```python
from build123d import *

# Parameters (mm, degrees)
F0_W     = 41.78606
F0_H     = 0.478756
F1_DEPTH = 1.5
F0_H_2   = 15.542488
F2_DEPTH = 1
F3_DEPTH = 1.5


with BuildPart() as f1:
    # F0 (on Right) → F1 (new body)
    with BuildSketch(Plane.YZ):
        with Locations((0, -8.010622)):
            Rectangle(F0_W, F0_H)
    extrude(amount=F1_DEPTH)

    # F0 (on Right) → F2 (join)
    with BuildSketch(Plane.YZ):
        with Locations((0, 8.010622)):
            Rectangle(F0_W, F0_H)
        Rectangle(F0_W, F0_H_2)
        with Locations((0, -8.010622)):
            Rectangle(F0_W, F0_H)
    extrude(amount=F2_DEPTH)

    # F0 (on Right) → F3 (join)
    with BuildSketch(Plane.YZ):
        with Locations((0, 8.010622)):
            Rectangle(F0_W, F0_H)
    extrude(amount=F3_DEPTH)


solid = f1.part
```
Design review of the part built by this model. Coordinates are the model's own, in mm. Coordinates: 2 decimals unless noted, no trailing zeros. Order: outer loops, then holes, each group sorted by start corner. A loop starts at its lowest first (then second) coordinate and runs counter-clockwise, first axis right, second up. Notation, with made-up numbers: M 11,-34 L 30,-34 A23 ccw 30,-24 Z; hole C 4,82 d9. An arc over 180 degrees is marked long. Answer as a JSON object with one key per item and string values. Group by question number.
1) Add section B-B, the plane y = -3.5. Write out the cut boundary in (x, z).
2) Add section C-C, the plane z = 7. Write out the cut boundary in (x, y), then the cut area to 3 significant figures.
3) Wall thickness on L1, parallel to Z at x = 1.1, y = 18; L2, parallel to X at y = 13, z = 4.5: over which ranges is each line inside the solid? List them lowest first.
4) Add section A-A, the plane x = 1.25. Write out the cut boundary in (y, z), then the cut area to 3 significant figures.
5) Mouldability with a two-part tool opening along Z and no side actions: class faces 1 (the flat face through (1, 0, -8.25)), 2 (the flat face through (1, 0, 8.25)), 3 (the flat face through (1, 0, 0)), 4 (the flat face through (0.4, -20.893, 0.1)) as pulls with the +Z half, pulls with the -Z half, needs draft (parallel to the pull), parting line crosses it, or undercut.
Computed values:
{
 "1": {"outline": "M 0,-8.25 L 1.5,-8.25 L 1.5,-7.77 L 1,-7.77 L 1,7.77 L 1.5,7.77 L 1.5,8.25 L 0,8.25 Z"},
 "2": {"outline": "M 0,-20.89 L 1,-20.89 L 1,20.89 L 0,20.89 Z", "area": "41.8 mm^2"},
 "3": {"L1": "z = -8.25 to -7.77, 7.77 to 8.25", "L2": "x = 0 to 1"},
 "4": {"outline": "M -20.89,-8.25 L 20.89,-8.25 L 20.89,-7.77 L -20.89,-7.77 Z; M -20.89,7.77 L 20.89,7.77 L 20.89,8.25 L -20.89,8.25 Z", "area": "40.0 mm^2"},
 "5": {"face 1": "pulls with the -Z half", "face 2": "pulls with the +Z half", "face 3": "undercut", "face 4": "needs draft"}
}
